Could you check a few things on this drawing? It's one solid part, dimensions in mm from its lowest x, y, z. A direction names the side the tool comes from. Coordinates: 2 decimals unless noted, no trailing zeros. Order: outer loops, then holes, each group sorted by start corner. A loop starts at its lowest first (then second) coordinate and runs counter-clockwise, first axis right, second up. Notation, with made-up numbers: M 13,-8.75 L 24,-8.75 A22 ccw 24,22.25 Z; hole C 10.5,48.25 d4. An arc over 180 degrees is marked long. One line per question, with ' | ' between items. Start each with the question number.
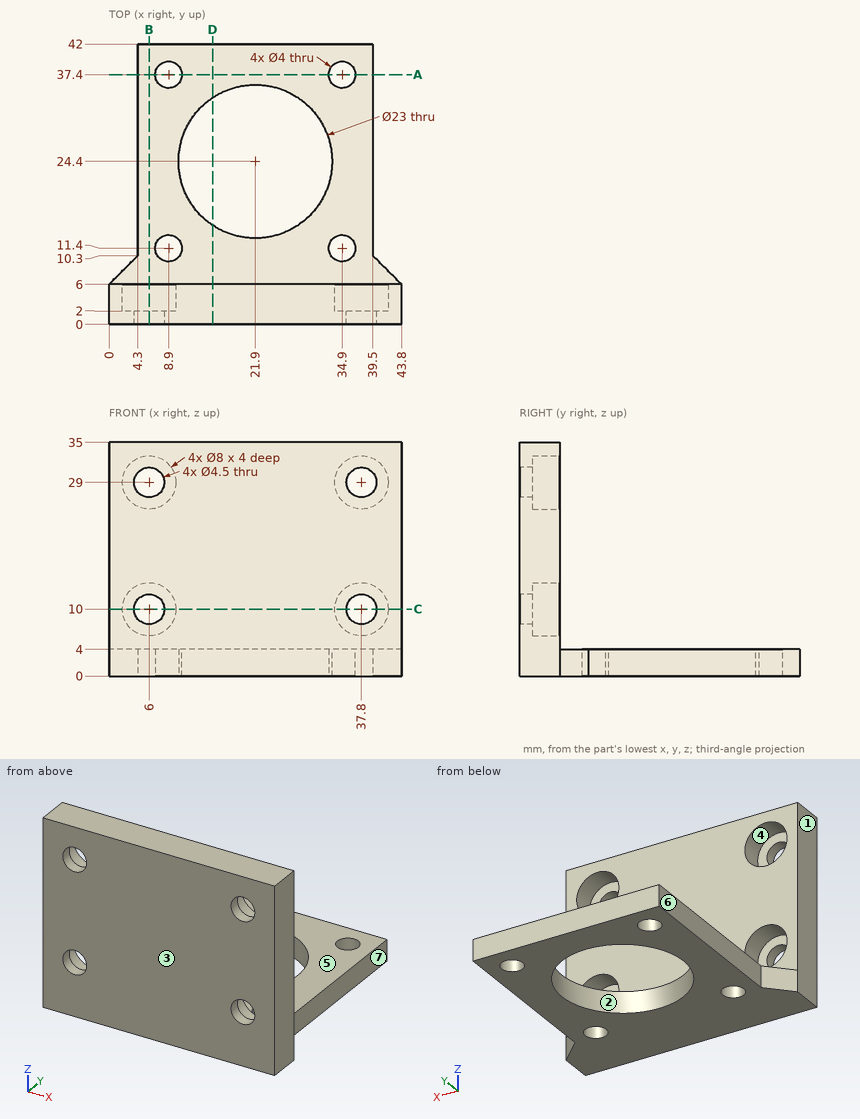
1. Will these pins go through, and if not, where does the flat tip stop? pin 1 (2.5 mm diameter, centred on x = 36, z = 28, fed in from +Y); pin 2 (6.5 mm diameter, centred on x = 5.5, z = 27.5, fed in from +Y); pin 3 (2 mm diameter, centred on y = 22, z = 2.5, fed in from +X).
2. We'd pull the mould along Y, two halves only. Please class the marked faces 1, 2 and 3: released by +Y, released by -Y, zero draft, split by the parting line, or undercut.
3. Which directions (+Z, -Z, +X, -X, +Y, -Y) give clear straight access to the entire face, cutting with the end or side of a thin tool? Please do the marked faces 4, 5, 6 and 7.
4. Imagine slicing it at C-C (z = 10). List the corners of the cut face in (x, y) for me, then the cut area to 3 significant figures.
5. I need wall thicknesses on line 1 (Z direction, x = 6, y = 3.1); line 2 (X direction, y = 5, z = 29); line 3 (Z direction, x = 7.5, y = 16). Which ranges of each line are inside material? Lowest first, please.
6. Imagine slicing it at B-B (x = 6). List the corners of the cut face in (y, z) for me.
7. Imagine slicing it at D-D (x = 15.5). List the corners of the cut face in (y, z) for me.
8. Imagine slicing it at A-A (y = 37.4). List the corners of the cut face in (x, z) for me.
Entries:
1) pin 1: y = 2 | pin 2: y = 6 | pin 3: x = 39.5
2) face 1: zero draft | face 2: undercut | face 3: released by -Y
3) face 4: +Y | face 5: +Z, +X, -X, +Y | face 6: +Z, -Z, -X, +Y | face 7: +Z, -Z, +X, +Y
4) outline: M 0,0 L 3.75,0 L 3.75,2 L 2,2 L 2,6 L 0,6 Z; M 8.25,0 L 35.55,0 L 35.55,2 L 33.8,2 L 33.8,6 L 10,6 L 10,2 L 8.25,2 Z; M 40.05,0 L 43.8,0 L 43.8,6 L 41.8,6 L 41.8,2 L 40.05,2 Z | area: 181 mm²
5) line 1: 0 to 6, 14 to 25, 33 to 35 | line 2: 0 to 2, 10 to 33.8, 41.8 to 43.8 | line 3: 0 to 4
6) outline: M 0,0 L 42,0 L 42,4 L 6,4 L 6,6 L 2,6 L 2,7.75 L 0,7.75 Z; M 0,12.25 L 2,12.25 L 2,14 L 6,14 L 6,25 L 2,25 L 2,26.75 L 0,26.75 Z; M 0,31.25 L 2,31.25 L 2,33 L 6,33 L 6,35 L 0,35 Z
7) outline: M 0,0 L 14.85,0 L 14.85,4 L 6,4 L 6,35 L 0,35 Z; M 33.95,0 L 42,0 L 42,4 L 33.95,4 Z
8) outline: M 4.3,0 L 6.9,0 L 6.9,4 L 4.3,4 Z; M 10.9,0 L 32.9,0 L 32.9,4 L 10.9,4 Z; M 36.9,0 L 39.5,0 L 39.5,4 L 36.9,4 Z
